Work out the finished part from the listing and answer in its coordinate system (mm). A direction names the side the tool comes from. Round coordinates to 2 decimals unless told otherwise and drop trailing zeros. Order: outer loops, then holes, each group sorted by start corner. A loop starts at its lowest first (then second) coordinate and runs counter-clockwise, first axis right, second up. Notation, with made-up numbers: (53, 80.25) - (92, 80.25) arc R34 cw to (92, 114.25) - close; hole circle Ø3 at (76.5, -33.5). An arc over 180 degrees is marked (long way). One line per question, with ' | ' between items. Start each with the question number.
from build123d import *

# Parameters (mm, degrees)
F4_DEPTH = 65
F5_DEPTH = 55
F6_DEPTH = 65.001
F7_DEPTH = 22
F8_DEPTH = 4


with BuildPart() as f3:
    # F2 (on Front) → F3 (revolve)
    with BuildSketch(Plane.XZ):
        Polygon((-65.5, 0), (0, 0), (0, 2), (-65.5, 6), align=None)
    revolve(axis=Axis((0, 0, 1), (0, 0, -1)))

    # F0 (on Top) → F4 (join)
    with BuildSketch(Plane.XY):
        with BuildLine():
            ThreePointArc((-50.175911, 42.102588), (19.076579, 62.660467), (65.12488, 7))
            Line((65.12488, 7), (64.31456, 7))
            ThreePointArc((64.31456, 7), (57.31456, 0), (64.31456, -7))
            Line((64.31456, -7), (65.12488, -7))
            ThreePointArc((65.12488, -7), (19.076579, -62.660467), (-50.175911, -42.102588))
            Line((-50.175911, -42.102588), (-51.708, -43.388164))
            ThreePointArc((-51.708, -43.388164), (20.719651, -64.241311), (67.31456, -5))
            Line((67.31456, -5), (64.31456, -5))
            ThreePointArc((64.31456, -5), (59.31456, 0), (64.31456, 5))
            Line((64.31456, 5), (67.31456, 5))
            ThreePointArc((67.31456, 5), (20.719651, 64.241311), (-51.708, 43.388164))
            Line((-51.708, 43.388164), (-50.175911, 42.102588))
        make_face()
    extrude(amount=F4_DEPTH)

    # F0 (on Top) → F5 (join)
    with BuildSketch(Plane.XY):
        with BuildLine():
            Line((-55.537341, -46.601363), (-51.708, -43.388164))
            ThreePointArc((-51.708, -43.388164), (-52.186928, -42.810916), (-52.659412, -42.228383))
            Line((-52.659412, -42.228383), (-56.489635, -45.442321))
            ThreePointArc((-56.489635, -45.442321), (-56.016486, -46.024305), (-55.537341, -46.601363))
        make_face()
        with BuildLine():
            ThreePointArc((-50.175911, -42.102588), (-65.5, 0), (-50.175911, 42.102588))
            Line((-50.175911, 42.102588), (-51.708, 43.388164))
            ThreePointArc((-51.708, 43.388164), (-52.186928, 42.810916), (-52.659412, 42.228383))
            ThreePointArc((-52.659412, 42.228383), (-67.5, 0), (-52.659412, -42.228383))
            ThreePointArc((-52.659412, -42.228383), (-52.186928, -42.810916), (-51.708, -43.388164))
            Line((-51.708, -43.388164), (-50.175911, -42.102588))
        make_face()
        with BuildLine():
            ThreePointArc((-52.659412, 42.228383), (-52.186928, 42.810916), (-51.708, 43.388164))
            Line((-51.708, 43.388164), (-55.537341, 46.601363))
            ThreePointArc((-55.537341, 46.601363), (-56.016486, 46.024305), (-56.489635, 45.442321))
            Line((-56.489635, 45.442321), (-52.659412, 42.228383))
        make_face()
    extrude(amount=F5_DEPTH)

    # F0 (on Top) → F6 (cut, through all)
    with BuildSketch(Plane.XY):
        with BuildLine():
            ThreePointArc((67.31456, -5), (67.5, 0), (67.31456, 5))
            Line((67.31456, 5), (64.31456, 5))
            ThreePointArc((64.31456, 5), (59.31456, 0), (64.31456, -5))
            Line((64.31456, -5), (67.31456, -5))
        make_face()
    extrude(amount=F6_DEPTH, mode=Mode.SUBTRACT)

    # F1 (on Top) → F7 (join)
    with BuildSketch(Plane.XY):
        with BuildLine():
            Line((6.545644, -2.5), (4.400658, -2.5))
            ThreePointArc((4.400658, -2.5), (20, 0), (4.400658, 2.5))
            Line((4.400658, 2.5), (6.545644, 2.5))
            ThreePointArc((6.545644, 2.5), (18, 0), (6.545644, -2.5))
        make_face()
    extrude(amount=F7_DEPTH)

    # F1 (on Top) → F8 (join)
    with BuildSketch(Plane.XY):
        with BuildLine():
            ThreePointArc((4.400658, 2.5), (20, 0), (4.400658, -2.5))
            Line((4.400658, -2.5), (1.287857, -2.5))
            ThreePointArc((1.287857, -2.5), (23, 0), (1.287857, 2.5))
            Line((1.287857, 2.5), (4.400658, 2.5))
        make_face()
    extrude(amount=F8_DEPTH)


solid = f3.part
1) Flat-ended cylindrical pins translate along their axes: pin 1 (4 mm diameter, centred on y = 24, z = 57.5, fed in from +X); pin 2 (8 mm diameter, centred on x = 14, y = 2.5, fed in from +Z); pin 3 (6 mm diameter, centred on x = -24.5, y = 1, fed in from +Z); pin 4 (14 mm diameter, centred on x = 12, y = 0, fed in from -Z). Find the tip coordinate at first contact, or state that the pin passes through.
2) Determine the mould class of faces 5 (the flat face through (-54.548, -43.813, 27.115)), 6 (the cylindrical face through (20, 0, 13)), 7 (the flat face through (-53.65, -45.02, 27.12)), 8 (the flat face through (60, 5, 65)) for opening direction Y: released by +Y, released by -Y, zero draft, split by the parting line, or undercut.
3) For faces 1 (the flat face through (-54.601, 43.858, 27.115)), 2 (the flat face through (5, -2.5, 12)), 3 (the cylindrical face through (19.651, -64.576, 32.045)), 4 (the flat face through (-53.596, 44.972, 27.115)), determine the directions among +Z, -Z, +X, -X, +Y, -Y from which every point of the face is accessible in a straight line to the end or side of a thin tool.
4) Section A-A on z = 52.5 is taken. Give the vertices of the cut face in (x, y), and give its area (3 significant figures).
5) Straight lines are drawn through the part: line 1 (X direction, y = 0, z = 8); line 2 (Y direction, x = 12, z = 13.5); line 3 (Y direction, x = 60, z = 61.5). For each, find the intervals that lie inside material, in ascending order.
Recorded:
1) pin 1: stops at x = 63.81 | pin 2: stops at z = 22 | pin 3: stops at z = 3.68 | pin 4: stops at z = 0
2) face 5: undercut | face 6: undercut | face 7: released by -Y | face 8: zero draft
3) face 1: +Z, -Z, -X | face 2: +Z | face 3: +Z, -Z, -Y | face 4: +Z, -Z, +Y
4) outline: (-56.49, -45.44) arc R72.5 ccw to (-55.54, -46.6) - (-51.71, -43.39) arc R67.5 ccw to (67.31, -5) - (64.31, -5) arc R5 cw to (64.31, 5) - (67.31, 5) arc R67.5 ccw to (-51.71, 43.39) - (-55.54, 46.6) arc R72.5 ccw to (-56.49, 45.44) - (-52.66, 42.23) arc R67.5 ccw to (-52.66, -42.23) - close; hole (-50.18, -42.1) arc R65.5 ccw to (65.12, -7) - (64.31, -7) arc R7 cw to (64.31, 7) - (65.12, 7) arc R65.5 ccw to (-50.18, 42.1) arc R65.5 ccw to start | area: 872 mm²
5) line 1: x = -67.5 to -65.5, 18 to 20, 57.31 to 59.31 | line 2: y = -66.42 to -64.39, -8 to -6, 6 to 8, 64.39 to 66.42 | line 3: y = -30.92 to -26.27, -5.51 to -2.53, 2.53 to 5.51, 26.27 to 30.92
